Build history of the part. All positions in model axes, mm. Face numbers are marked on the shaded views. A direction names the side the tool comes from. Give positions to 0.01 mm unless a question says otherwise; leave off trailing zeros. Order: outer loops, then holes, each group sorted by start corner. A loop starts at its lowest first (then second) coordinate and runs counter-clockwise, first axis right, second up. Notation, with made-up numbers: (-33, 44) -> (-13, 44) arc R28 ccw to (-13, 75) -> close; hole circle Ø1 at (7.25, 72). An arc over 180 degrees is marked (long way). One line per item, written item: value. Start each with the question number.
(1) Probe line 1 (Z direction, x = -27, y = 11.5); line 2 (Y direction, x = 24.5, z = 15) (3 decimals); line 3 (X direction, y = 1, z = -8). List the from-to ranges inside material, lowest first.
(2) Saw through at C-C on z = 28. Give the cut face in (x, y).
(3) Pin check, flat tips, straight feed: pin 1 (2 mm diameter, centred on x = -12.5, z = 37, fed in from -Y); pin 2 (1 mm diameter, centred on x = -15, z = 6, fed in from +Y); pin 3 (6 mm diameter, centred on x = -23.5, z = -1.5, fed in from -Y); pin 4 (1 mm diameter, centred on x = -16.5, z = 12.5, fed in from -Y). Stop position of each tip, or through.
(4) Saw through at D-D on z = -18. Give the cut face in (x, y), plus the area to 3 significant figures.
(5) Saw through at A-A on x = 0. Give the cut face in (y, z), plus the area to 3 significant figures.
(6) Which spindle directions (+Z, -Z, +X, -X, +Y, -Y) get a long thin tool onto all of the face, cutting with end or side? Do the marked faces 1, 2 and 3. Say none if no direction does.
Autodesk Fusion 360 part; units mm, degrees
sketch "Sketch1" plane through (0, 0, 0) normal (0, 0, 1) x (1, 0, 0)
  circle A0 centre (0, 0) radius 35
  dimension "d1" = 70
extrude "Extrude1" add sketch "Sketch1" along normal blind 25
sketch "Sketch2" plane through (0, 0, 25) normal (0, 0, 1) x (-1, 0, 0)
  circle A0 centre (0, 0) radius 35
  circle A1 centre (0, 0) radius 10
  dimension "d4" = 20
extrude "Extrude2" add sketch "Sketch2" along normal blind 25 contours A1
mirror "Mirror1" about plane through (0, 0, 0) normal (0, 0, 1) of bodies 1 merged
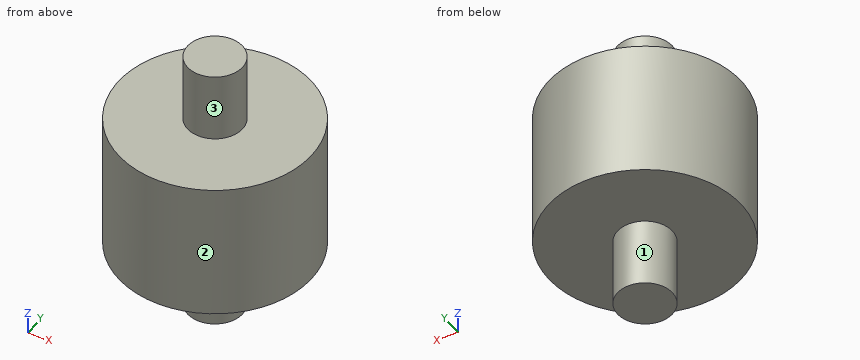
Results below:
1. line 1: z = -25 to 25
1. line 2: y = -24.995 to 24.995
1. line 3: x = -34.99 to 34.99
2. outline: circle Ø20 at (0, 0)
3. pin 1: passes through
3. pin 2: stops at y = 31.86
3. pin 3: stops at y = -28.37
3. pin 4: stops at y = -31.13
4. outline: circle Ø70 at (0, 0)
4. area: 3,850 mm²
5. outline: (-35, -25) -> (-10, -25) -> (-10, -50) -> (10, -50) -> (10, -25) -> (35, -25) -> (35, 25) -> (10, 25) -> (10, 50) -> (-10, 50) -> (-10, 25) -> (-35, 25) -> close
5. area: 4,500 mm²
6. face 1: -Z
6. face 2: +Z, -Z
6. face 3: +Z
